Geometry check sheet. Reference: the model listing, model coordinates, mm. Face numbers are marked on the shaded views. Give positions to 0.01 mm unless a question says otherwise; leave off trailing zeros. Order: outer loops, then holes, each group sorted by start corner. A loop starts at its lowest first (then second) coordinate and runs counter-clockwise, first axis right, second up.
```python
from build123d import *


with BuildPart() as part:
    # Sketch2 → Revolve1 (revolve)
    with BuildSketch(Plane.XY, mode=Mode.PRIVATE) as revolve1_sk:
        with BuildLine():
            Line((0, 0), (-11.96988083, 0))
            Line((-11.96988083, 0), (-11.96988083, 1.340283376))
            ThreePointArc((-11.96988083, 1.340283376), (-11.2331295, 1.901248909), (-10.404461542, 2.314521541))
            ThreePointArc((-10.404461542, 2.314521541), (-11.106179845, 2.880731417), (-11.63207258, 3.613151399))
            ThreePointArc((-11.63207258, 3.613151399), (-11.670741013, 4.017061246), (-11.412476332, 4.330011348))
            Line((-11.412476332, 4.330011348), (-8.737098944, 6.352490289))
            ThreePointArc((-8.737098944, 6.352490289), (-8.132098156, 6.91410221), (-7.651964701, 7.585597383))
            ThreePointArc((-7.651964701, 7.585597383), (-7.094925104, 8.174757479), (-6.330073896, 8.443839921))
            ThreePointArc((-6.330073896, 8.443839921), (-4.606295289, 13.210063627), (-4.021311984, 18.244554231))
            Line((-4.021311984, 18.244554231), (-4.021311984, 21.208163842))
            ThreePointArc((-4.021311984, 21.208163842), (-5.580309883, 21.442384278), (-7.115742629, 21.799847488))
            ThreePointArc((-7.115742629, 21.799847488), (-7.325805309, 22.03138024), (-7.205776672, 22.320044181))
            ThreePointArc((-7.205776672, 22.320044181), (-5.06963874, 23.609952102), (-2.778232272, 24.598083726))
            Line((-2.778232272, 24.598083726), (-2.778232272, 24.845430157))
            ThreePointArc((-2.778232272, 24.845430157), (-6.247093969, 32.04409144), (0, 37.026815862))
            Line((0, 37.026815862), (0, 0))
        make_face()
    revolve(revolve1_sk.sketch.rotate(Axis((0, 0, 0), (0, 1, 0)), 270), axis=Axis((0, 0, 0), (0, 1, 0)))


solid = part.part
```
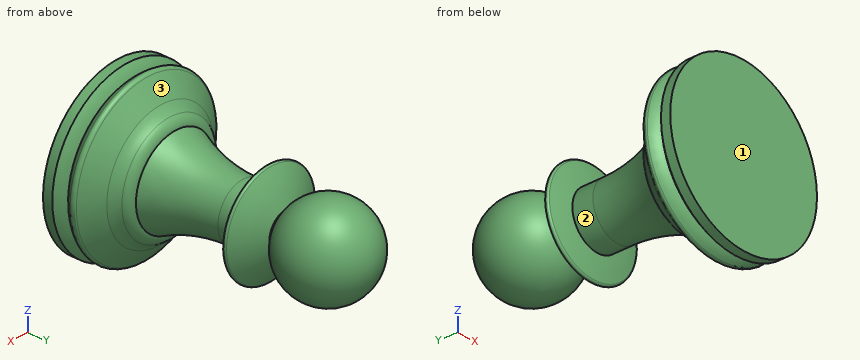
Q1. Cross-section at A-A, the plane y = 10. Record the boundary of the cut face in (x, z), and give its area (3 significant figures).
Q2. Gauge pin test, flat ends, axial feed: P1, Ø6, axis at x = 5, y = 22, coming from the +Z side; P2, Ø8, axis at x = -5, y = 5, coming from the -Z side; P3, Ø1.5, axis at y = 28.5, z = 6, coming from the -X side; P4, Ø4, axis at x = 9.5, y = 27.5, coming from the -Z side. Record the tip position at first contact, or that the pin passes through.
Q3. Thickness scan on L1, parallel to Y at x = 3, z = 4.25; L2, parallel to Y at x = -5.5, z = -9; L3, parallel to Y at x = -10, z = -3.5. Record the ranges inside material, lowest first.
Q4. Release check for a two-part mould opening along Y. For the marked faces 1, 2 and 3 record: pulls with the +Y half, pulls with the -Y half, needs draft (parallel to the pull), parting line crosses it, or undercut.
Q5. Cross-section at B-B, the plane y = 16.5. Record the boundary of the cut face in (x, z), and give its area (3 significant figures).
Answers follow:
1. outline: circle Ø11.26 at (0, 0)
1. area: 99.5 mm2
2. P1: stops at z = 7.05
2. P2: stops at z = -11.64
2. P3: stops at x = -3.09
2. P4: passes through
3. L1: y = 0 to 11.14, 21.37 to 23.54, 26.88 to 34.36
3. L2: y = 0 to 2.26, 2.41 to 4.98
3. L3: y = 0 to 2.24, 2.44 to 4.95
4. face 1: pulls with the -Y half
4. face 2: undercut
4. face 3: pulls with the +Y half
5. outline: circle Ø8.18 at (0, 0)
5. area: 52.6 mm2
